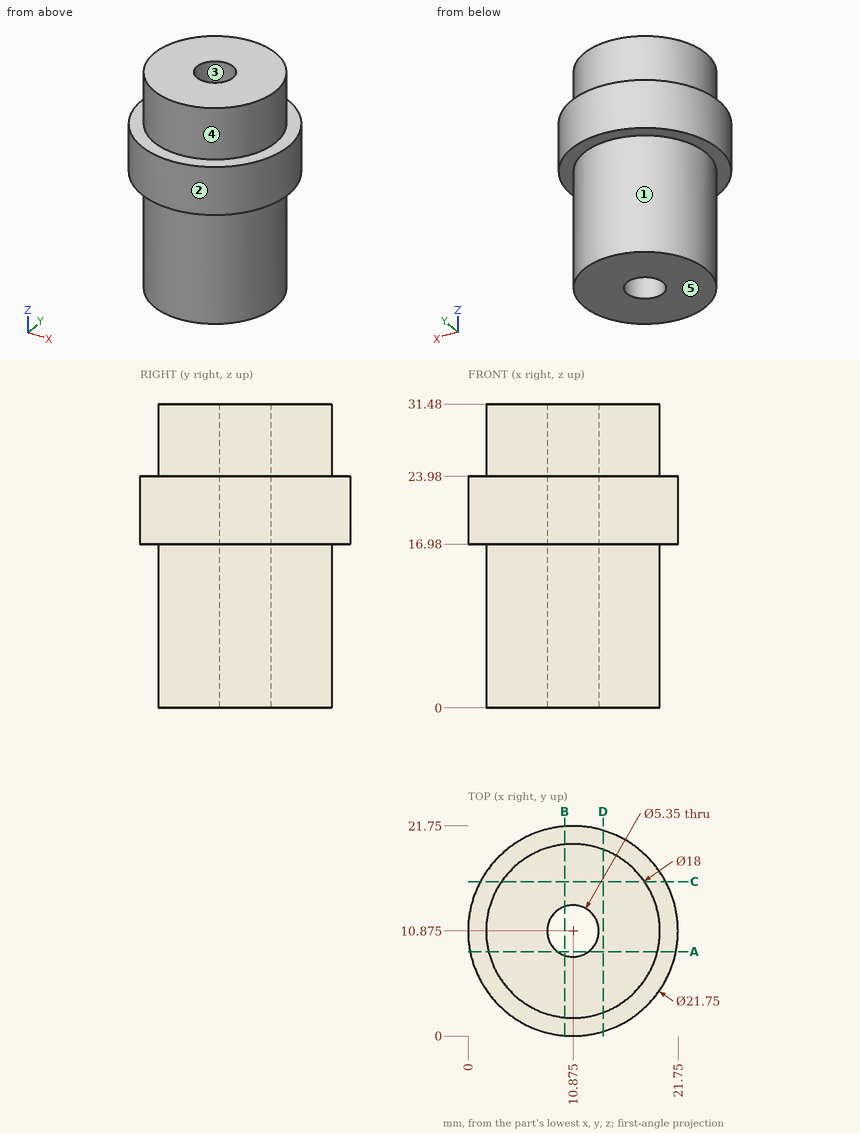
Job drawing, mm, ordinate dimensions from the low corner. One solid piece. A direction names the side the tool comes from. Round coordinates to 2 decimals unless told otherwise and drop trailing zeros. Write each loop counter-clockwise with the first axis right and the second up, starting at its lowest first coordinate (ties: lowest second). Pieces come first, ordered by that corner, then holes. Notation, with made-up numbers: M 83,3.25 L 121,3.25 A18 cw 121,16.25 Z; hole C -16.75,43.25 d2. An arc over 180 degrees is marked long. Return JSON: item names as keys, results as strings. Group by question number.
(1) Drill centre lines: probe 1 along X at (y, z) = (10.75, 28.5); probe 2 along X at (y, z) = (13, 11); probe 3 along Z at (x, y) = (2, 15.75). Where is each one in solid material? Low to high.
(2) Saw through at A-A on y = 8.75. Write the cut outline in (x, z), then the cut area to 3 significant figures.
(3) Pin check, flat tips, straight feed: pin 1 Ø2 at (x, z) = (19.5, 26) entering from -Y; pin 2 Ø3 at (y, z) = (3.5, 26.5) entering from +X; pin 3 Ø4.5 at (x, y) = (10.875, 10.875) entering from +Z; pin 4 Ø6 at (y, z) = (13, 12.5) entering from +X (3 decimals). Stop position of each tip, or through.
(4) Saw through at C-C on y = 16. Write the cut outline in (x, z).
(5) Which spindle directions (+Z, -Z, +X, -X, +Y, -Y) get a long thin tool onto all of the face, cutting with end or side? Do the marked faces 1 and 2. Say none if no direction does.
(6) Saw through at D-D on x = 14. Write the cut outline in (y, z), then the cut area to 3 significant figures.
(7) Saw through at B-B on x = 10. Write the cut outline in (y, z), then the cut area to 3 significant figures.
(8) Two-plate mould, pull along Y, no slides. Class the marked faces 3, 4 and 5: +Y half, -Y half, draft (parallel to the pull), parting line (faces both ways), or undercut.
Returned:
{
 "1": {"probe 1": "1.88 to 8.2, 13.55 to 19.87", "probe 2": "2.13 to 9.25, 12.5 to 19.62", "probe 3": "16.98 to 23.98"},
 "2": {"outline": "M 0.21,16.98 L 2.13,16.98 L 2.13,0 L 9.25,0 L 9.25,31.48 L 2.13,31.48 L 2.13,23.98 L 0.21,23.98 Z; M 12.5,0 L 19.62,0 L 19.62,16.98 L 21.54,16.98 L 21.54,23.98 L 19.62,23.98 L 19.62,31.48 L 12.5,31.48 Z", "area": "475 mm²"},
 "3": {"pin 1": "y = 6.09", "pin 2": "x = 17.69", "pin 3": "through", "pin 4": "x = 19.875"},
 "4": {"outline": "M 1.28,16.98 L 3.48,16.98 L 3.48,0 L 18.27,0 L 18.27,16.98 L 20.47,16.98 L 20.47,23.98 L 18.27,23.98 L 18.27,31.48 L 3.48,31.48 L 3.48,23.98 L 1.28,23.98 Z"},
 "5": {"face 1": "-Z", "face 2": "+Z, -Z"},
 "6": {"outline": "M 0.46,16.98 L 2.43,16.98 L 2.43,0 L 19.32,0 L 19.32,16.98 L 21.29,16.98 L 21.29,23.98 L 19.32,23.98 L 19.32,31.48 L 2.43,31.48 L 2.43,23.98 L 0.46,23.98 Z", "area": "559 mm²"},
 "7": {"outline": "M 0.04,16.98 L 1.92,16.98 L 1.92,0 L 8.35,0 L 8.35,31.48 L 1.92,31.48 L 1.92,23.98 L 0.04,23.98 Z; M 13.4,0 L 19.83,0 L 19.83,16.98 L 21.71,16.98 L 21.71,23.98 L 19.83,23.98 L 19.83,31.48 L 13.4,31.48 Z", "area": "431 mm²"},
 "8": {"face 3": "undercut", "face 4": "parting line", "face 5": "draft"}
}
